Can you work these out from the model? Positions are in its coordinate system, mm. A direction names the side the tool comes from. Coordinates: 2 decimals unless noted, no trailing zeros. Order: outer loops, then holes, each group sorted by start corner. A loop starts at its lowest first (then second) coordinate and runs counter-clockwise, first axis right, second up.
```python
from build123d import *

# Parameters (mm, degrees)
F0_R     = 12.5
F0_R_2   = 6
F1_DEPTH = 25
F2_DEPTH = 25
F4_R     = 7.5


with BuildPart() as f1:
    # F0 (on Top) → F1 (new body)
    with BuildSketch(Plane.XY):
        Circle(F0_R)
        Circle(F0_R_2, mode=Mode.SUBTRACT)
    extrude(amount=F1_DEPTH)



with BuildPart() as f2:
    # F0 (on Top) → F2 (new body)
    with BuildSketch(Plane.XY):
        with Locations((150, 0)):
            Circle(F0_R)
        with Locations((150, 0)):
            Circle(F0_R_2, mode=Mode.SUBTRACT)
    extrude(amount=-F2_DEPTH)


with BuildPart() as f1_1:
    add(f1.part)

    add(f2.part)  # F5 merges F2
    # F5: sweep along a path in F3
    with BuildLine(Plane.XZ) as f5_path:
        Line((0, 12), (25, 12))
        ThreePointArc((25, 12), (73.4611796798, -6.6552812809), (125, -13))
        Line((125, -13), (150, -13))
    # F4 (on Right) → F5 (sweep)
    with BuildSketch(Plane.YZ):
        with Locations((0, 12)):
            Circle(F4_R)
    sweep(path=f5_path.line, transition=Transition.RIGHT)


solid = f1_1.part
```
1. Imagine slicing it at B-B on y = 0. Give the number of separate pieces and of enclosed holes in the cut face, then the cut area to 3 significant figures.
Completed:
separate pieces: 3
enclosed holes: 0
area: 2,770 mm2
2. I'm going to push flat-ended pins straight in: pin 1 (8 mm diameter, centred on x = 132.5, y = 9.5, fed in from -Z); pin 2 (12 mm diameter, centred on x = 23.5, z = -6, fed in from -Y); pin 3 (5 mm diameter, centred on x = 71, y = -4, fed in from +Z); pin 4 (12.5 mm diameter, centred on x = 2.5, y = -3, fed in from -Z). Where does each tip first touch, or does it pass through?
Completed:
pin 1: stops at z = -18.1
pin 2: passes through
pin 3: stops at z = 1.88
pin 4: stops at z = 0
3. Please list where these lines run through material, in increasing order: probe 1 along Z at (x, y) = (2, -10.75); probe 2 along X at (y, z) = (2.75, -21); probe 3 along X at (y, z) = (1, 19.5).
Completed:
probe 1: z = 0 to 25
probe 2: x = 137.81 to 144.67, 155.33 to 162.19
probe 3: x = -12.46 to -5.92, 5.92 to 12.46
4. On a 3-axis mill with a long thin cutter (end or side, diameter ignored), from which of +Z, -Z, +X, -X, +Y, -Y can I reach the whole of each face in a straight line? I mean faces 4 (the flat face through (150, 0, -13)), 5 (the cylindrical face through (-6, 0, 12)), 6 (the flat face through (-3, -5.4, 25)), 7 (the flat face through (-3, -5.4, 0)), 8 (the flat face through (155.4, 3, 0)). Say none if no direction works.
Completed:
face 4: +Z, -Z
face 5: none
face 6: +Z, +X, -X, +Y, -Y
face 7: -Z, -X, +Y, -Y
face 8: +Z, +X, +Y, -Y
5. Imagine slicing it at A-A on y = 9.75. Please give me the cut outline in (x, z).
Completed:
outline: (-7.82, 0) - (7.82, 0) - (7.82, 25) - (-7.82, 25) - close; (142.18, -25) - (157.82, -25) - (157.82, 0) - (142.18, 0) - close
6. Thinking about a two-plate mould opening in Y: for faces 1 (the flat face through (0, 0, 12)), 2 (the cylindrical face through (18.556, -0.976, 19.436)), 3 (the flat face through (155.4, 3, -25)), which applies, pulls with the +Y half, pulls with the -Y half, needs draft (parallel to the pull), parting line crosses it, or undercut?
Completed:
face 1: undercut
face 2: parting line crosses it
face 3: needs draft
7. Imagine slicing it at C-C on y = -10.25. Please give me the cut outline in (x, z).
Completed:
outline: (-7.15, 0) - (7.15, 0) - (7.15, 25) - (-7.15, 25) - close; (142.85, -25) - (157.15, -25) - (157.15, 0) - (142.85, 0) - close
